from build123d import *

# Parameters (mm, degrees)
F1_DEPTH      = 2
F1_DEPTH_BACK = 2
F2_R          = 1
F3_DEPTH      = 2


with BuildPart() as f1:
    # F0 (on Top) → F1 (new body, two sides)
    with BuildSketch(Plane.XY) as f1_sk:
        Polygon((6, 0), (-6, 0), (-6, 50), (-25, 50), (-25, 0), (-20, 0), (-20, -100), (170, -100), (170, 0), (175, 0), (175, 50), (156, 50), (156, 0), (144, 0), (144, 50), (83, 50), (83, 40), (95, 40), (95, 32), (85, 32), (85, 0), (105, 0), (105, -70), (45, -70), (45, 0), (65, 0), (65, 32), (55, 32), (55, 40), (67, 40), (67, 50), (6, 50), align=None)
    extrude(amount=F1_DEPTH)
    extrude(f1_sk.sketch, amount=-F1_DEPTH_BACK)

    # F2 (on face) → F3 (join)
    with BuildSketch(Plane(origin=(0, 0, 0), x_dir=(-1, 0, 0), z_dir=(0, 1, 0))):
        with Locations((-150, 0)):
            Circle(F2_R)
        Circle(F2_R)
    extrude(amount=F3_DEPTH)


solid = f1.part
Geometry check sheet. Reference: the model listing, model coordinates, mm. A direction names the side the tool comes from. Give positions to 0.01 mm unless a question says otherwise; leave off trailing zeros. Write each loop counter-clockwise with the first axis right and the second up, starting at its lowest first coordinate (ties: lowest second). Pieces come first, ordered by that corner, then holes. Notation, with made-up numbers: M 83.25,-15 L 119.25,-15 A29 cw 119.25,6 Z; hole C 71,69 d8. An arc over 180 degrees is marked long. Answer as CSV lines item,"result". Start each with the question number.
Q1. Go/stop test with flat-tipped pins: pin 1 (1.2 mm diameter, centred on x = -2.5, z = 0.5, fed in from +Y); pin 2 (1.5 mm diameter, centred on y = -22.5, z = -1.5, fed in from +X). Record where each tip stops, or that it passes through.
Q2. Tool access check on faces 1 (the face through (45, -35, 0)), 2 (the face through (-23, 0, 0)), 3 (the face through (144, 25, 0)). Record the directions out of +Z, -Z, +X, -X, +Y, -Y that give a thin tool (end or side, any length) a straight path to the whole face; none if there is none.
Q3. Section check A-A, the plane y = 4.5. Record the cut outline in (x, z), then the cut area to 3 significant figures.
Q4. Section check D-D, the plane x = 75. Record the cut outline in (y, z), then the cut area to 3 significant figures.
Q5. Material ranges on L1, parallel to X at y = 28, z = 1.3; L2, parallel to Y at x = 64.5, z = -0.8; L3, parallel to X at y = -24.5, z = -1.05, recorded low to high.
Q6. Section check C-C, the plane y = -41. Record the cut outline in (x, z).
Q7. Release check for a two-part mould opening along X. For faces 4 (the face through (166, 50, 0)), 5 (the face through (170, -51, 0)), 6 (the face through (90, 32, 0)) record: pulls with the +X half, pulls with the -X half, needs draft (parallel to the pull), parting line crosses it, or undercut.
Q8. Section check B-B, the plane x = 101. Record the cut outline in (y, z), then the cut area to 3 significant figures.
Geometry says:
1,pin 1,"y = 0"
1,pin 2,"x = 170"
2,face 1,"+Z, -Z"
2,face 2,"+Z, -Z, -X, -Y"
2,face 3,"+Z, -Z, +Y"
3,outline,"M -25,-2 L -6,-2 L -6,2 L -25,2 Z; M 6,-2 L 65,-2 L 65,2 L 6,2 Z; M 85,-2 L 144,-2 L 144,2 L 85,2 Z; M 156,-2 L 175,-2 L 175,2 L 156,2 Z"
3,area,"624 mm^2"
4,outline,"M -100,-2 L -70,-2 L -70,2 L -100,2 Z"
4,area,"120 mm^2"
5,L1,"-25 to -6, 6 to 65, 85 to 144, 156 to 175"
5,L2,"-100 to -70, 0 to 32, 40 to 50"
5,L3,"-20 to 45, 105 to 170"
6,outline,"M -20,-2 L 45,-2 L 45,2 L -20,2 Z; M 105,-2 L 170,-2 L 170,2 L 105,2 Z"
7,face 4,"needs draft"
7,face 5,"pulls with the +X half"
7,face 6,"undercut"
8,outline,"M -100,-2 L -70,-2 L -70,2 L -100,2 Z; M 0,-2 L 50,-2 L 50,2 L 0,2 Z"
8,area,"320 mm^2"
